Autodesk Inventor part; units mm, degrees
ref_plane "YZ Plane" through (0, 0, 0) normal (1, 0, 0) x (0, 1, 0)
ref_plane "XZ Plane" through (0, 0, 0) normal (0, 1, 0) x (-1, 0, 0)
ref_plane "XY Plane" through (0, 0, 0) normal (0, 0, 1) x (1, 0, 0)
sketch "Sketch1" plane through (0, 0, 0) normal (0, 1, 0) x (-1, 0, 0)
  arc A0 (50.8, 0) -> (4.3366, 50.6146) centre (0, 0) ccw
  line L0 (3.175, 51.8799) -> (3.175, 60.2257)
  line L1 (0, 60.2257) -> (0, 48.8785)
  arc A1 (47.625, 0) -> (1.237, 47.6089) centre (0, 0) ccw
  line L2 (3.175, 60.2257) -> (0, 60.2257)
  line L3 (50.8, 0) -> (47.6207, 0)
  line L4 (0, 47.625) -> (0, -34.2701) construction
  line L5 (50.8, 0) -> (0, 0) construction
  arc A2 (3.175, 51.8799) -> (4.3366, 50.6146) centre (4.445, 51.8799) ccw
  arc A3 (0, 48.8785) -> (1.237, 47.6089) centre (1.27, 48.8785) ccw
  point P0 (3.175, 50.7007)
  dimension "d5" = 3.175
  dimension "d20" = 3.175
  dimension "d22" = 9.525
  dimension "d23" = 50.8
  dimension "d24" = 1.27
revolve "Revolution1" add sketch "Sketch1" angle 360 about axis through (-50.8, 0, 0) along (1, 0, 0)
sketch "Sketch2" plane through (-3.175, 0, 0) normal (-1, 0, 0) x (0, 0, 1)
  circle A0 centre (0, 55.245) radius 1.4986
  circle A1 centre (0, 0) radius 50.7007
  circle A2 centre (-47.8436, 27.6225) radius 1.4986
  circle A3 centre (-47.8436, -27.6225) radius 1.4986
  circle A4 centre (0, -55.245) radius 1.4986
  circle A5 centre (47.8436, -27.6225) radius 1.4986
  circle A6 centre (47.8436, 27.6225) radius 1.4986
  point P0 (0, 0)
  dimension "d10" = 2.9972
  dimension "d12" = 55.245
  dimension "d15" = 360
extrude "Extrusion1" cut sketch "Sketch2" against normal blind 254 contours A0 | A2 | A3 | A4 | A5 | A6
properties part number "ROV Dome 4''"
Check sheet for the modelled part. Datum: model origin and axes. Units: mm. A direction names the side the tool comes from. Round coordinates to 2 decimals unless told otherwise and drop trailing zeros. Answer as a JSON object with one key per item and string values.
1. Mould release check, pull along Y, two halves, no side actions. Record for faces 3 (the cylindrical face through (-1.61, -28.95, -47.15)), 4 (the flat face through (0, 49, -5)), 5 (the cylindrical face through (-1.565, -59.713, -7.84)): pulls with the +Y half, pulls with the -Y half, needs draft (parallel to the pull), parting line crosses it, or undercut.
Reply:
{"face 3": "undercut", "face 4": "needs draft", "face 5": "parting line crosses it"}
2. Gauge pin test, flat ends, axial feed: P1, Ø3.5, axis at y = 27.62, z = -47.84, coming from the -X side (3 decimals); P2, Ø12, axis at x = -28.5, z = 41.5, coming from the -Y side; P3, Ø10, axis at y = 8.5, z = 25, coming from the -X side. Record the tip position at first contact, or that the pin passes through.
Reply:
{"P1": "stops at x = -3.175", "P2": "stops at y = -24.78", "P3": "stops at x = -46.07"}
3. Scan lines: line 1 (X direction, y = -35.5, z = 41) (3 decimals); line 2 (Y direction, x = -2, z = 0); line 3 (Z direction, x = -7.5, y = -24). Record each from-to range of solid material in increasing order.
Reply:
{"line 1": "x = -3.175 to 0", "line 2": "y = -60.23 to -56.74, -53.75 to -47.58, 47.58 to 53.75, 56.74 to 60.23", "line 3": "z = -44.14 to -40.45, 40.45 to 44.14"}
4. Access from +Z, -Z, +X, -X, +Y, -Y to the whole of each face (thin tool, end or side, straight path). Record for faces 1 (the flat face through (-3.175, -45, -27)), 2 (the cylindrical face through (-1.61, 53.915, 0.692)).
Reply:
{"face 1": "-X", "face 2": "+X, -X"}
